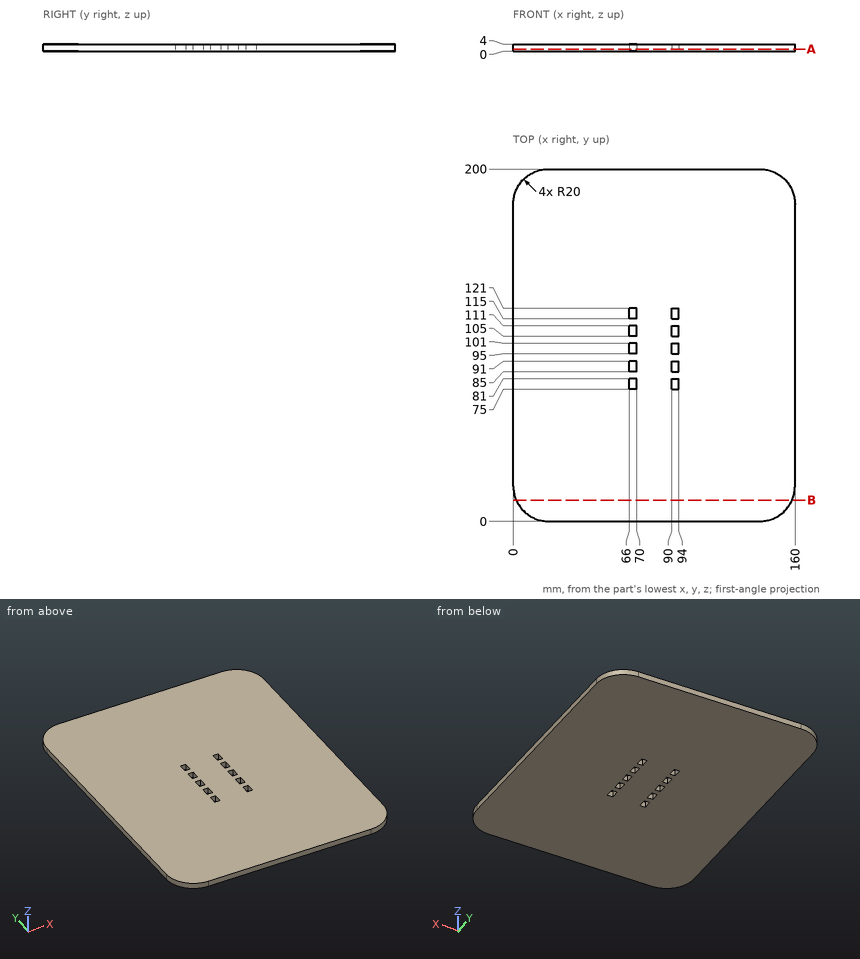
The drawing under review shows one solid part. Ordinate dimensions are in mm from its lowest x, y, z. Give positions to 0.01 mm unless a question says otherwise; leave off trailing zeros. Loops run counter-clockwise (first coordinate to the right, second up) from the corner with the lowest first, then second, coordinate; pieces in that order, holes last. Notation, with made-up numbers: M -32,55 L 12,55 A26 cw 12,69 Z; hole C 57.5,60.5 d11. An arc over 180 degrees is marked long. One line per item, written item: value. Start each with the question number.
Q1. For L1, parallel to X at y = 107, z = 2.35; L2, parallel to Y at x = 67.5, z = 0.75; L3, parallel to Y at x = 146, z = 3.3, list the stretches that pass through material, from the lowest coordinate up.
Q2. Add section B-B (y = 12). Give the boundary of the cut face in (x, z).
Q3. Add section A-A (z = 1.15). Count the separate pieces of the cut face and the enclosed holes in it, and give its area (3 significant figures).
Reply:
1. L1: 0 to 66, 70 to 90, 94 to 160
1. L2: 0 to 75, 81 to 85, 91 to 95, 101 to 105, 111 to 115, 121 to 200
1. L3: 0.92 to 199.08
2. outline: M 1.67,0 L 158.33,0 L 158.33,4 L 1.67,4 Z
3. separate pieces: 1
3. enclosed holes: 10
3. area: 31,400 mm²
